Geometry check sheet. Reference: the model listing, model coordinates, mm. Face numbers are marked on the shaded views. A direction names the side the tool comes from. Round coordinates to 2 decimals unless told otherwise and drop trailing zeros. Loops run counter-clockwise (first coordinate to the right, second up) from the corner with the lowest first, then second, coordinate; pieces in that order, holes last.
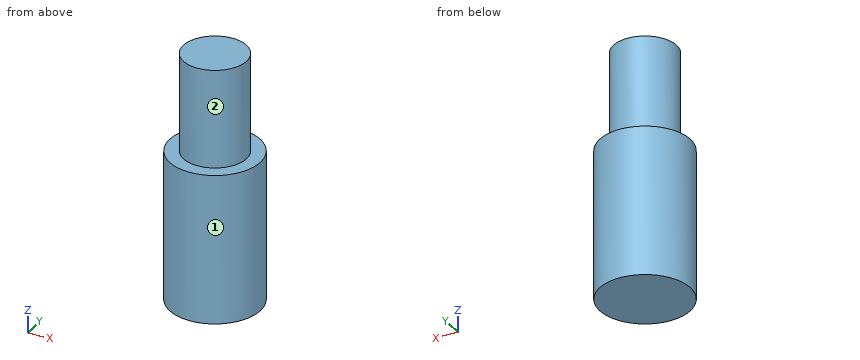
```python
from build123d import *

# Parameters (mm, degrees)
F0_W     = 32.885318622
F0_H     = 108.601231128
F2_T     = -10
F3_DEPTH = 170


with BuildPart() as f1:
    # F0 (on Front) → F1 (revolve)
    with BuildSketch(Plane.XZ):
        with Locations((-16.4426611736, -4.2723771185)):
            Rectangle(F0_W, F0_H)
    revolve(axis=Axis((-1.8626e-06, 0, -4.2723771185), (0, 0, -1)))

    # F2
    f2_openings = [f1.faces().sort_by_distance(p)[0] for p in [
        (-2e-06, 0, 50.028238),
    ]]
    offset(amount=F2_T, openings=f2_openings)

    # F3 (add): a face of the model
    f3_faces = [f1.faces().sort_by_distance(p)[0] for p in [
        (-1.8626e-06, 0, -48.5729926825),
    ]]
    extrude(f3_faces, amount=F3_DEPTH)


solid = f1.part
```
1) Scan lines: line 1 along Z through (x, y) = (19, -19); line 2 along Y through (x, z) = (1.5, -36); line 3 along X through (y, z) = (8.5, 57). Record each from-to range of solid material in increasing order.
Report:
line 1: z = -58.57 to 50.03
line 2: y = -32.85 to 32.85
line 3: x = -21.25 to 21.25
2) Sectioned sample at B-B, the plane x = -19. Record the cut outline in (y, z).
Report:
outline: (-26.84, -58.57) - (26.84, -58.57) - (26.84, 50.03) - (12.76, 50.03) - (12.76, 121.43) - (-12.76, 121.43) - (-12.76, 50.03) - (-26.84, 50.03) - close
3) Sectioned sample at C-C, the plane z = 10. Record the cut outline in (x, y), then the cut area to 3 significant figures.
Report:
outline: circle Ø65.77 at (0, 0)
area: 3,400 mm2
4) Access from +Z, -Z, +X, -X, +Y, -Y to the whole of each face (thin tool, end or side, straight path). Record for the marked faces 1 and 2.
Report:
face 1: +Z, -Z
face 2: +Z
5) Gauge pin test, flat ends, axial feed: pin 1 (3 mm diameter, centred on y = 2.5, z = -3.5, fed in from -X); pin 2 (10 mm diameter, centred on x = 19.5, z = 7, fed in from +Y); pin 3 (8 mm diameter, centred on x = -19.5, y = -26, fed in from +Z). Record the tip position at first contact, or that the pin passes through.
Report:
pin 1: stops at x = -32.87
pin 2: stops at y = 29.52
pin 3: stops at z = 50.03
6) Sectioned sample at D-D, the plane z = 56. Record the cut outline in (x, y).
Report:
outline: circle Ø45.77 at (0, 0)
7) Sectioned sample at A-A, the plane y = 0. Record the cut outline in (x, z).
Report:
outline: (-32.89, -58.57) - (32.89, -58.57) - (32.89, 50.03) - (22.89, 50.03) - (22.89, 121.43) - (-22.89, 121.43) - (-22.89, 50.03) - (-32.89, 50.03) - close
